Geometry: see drawing. Coordinates: mm, zero at the bounding-box minimum. Round coordinates to 2 decimals unless told otherwise and drop trailing zeros. Order: outer loops, then holes, each group sorted by start corner. A loop starts at its lowest first (then second) coordinate and runs counter-clockwise, first axis right, second up. Notation, with made-up numbers: (16.25, 50) -> (72.25, 50) arc R20 ccw to (72.25, 62) -> close; hole circle Ø8 at (51, -15). An arc over 180 degrees is marked (long way). Use a Markdown table: item, result.
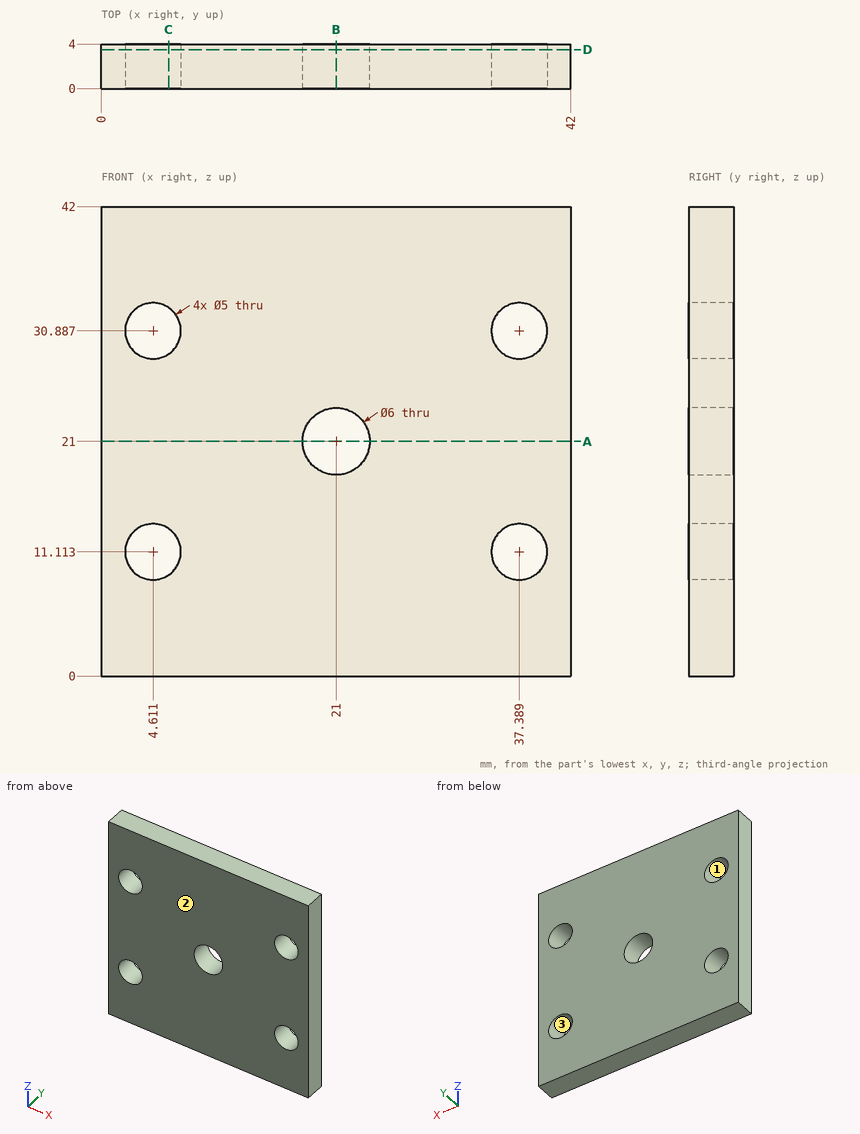
1) Cut plane A-A on z = 21. Return loops of the section in (x, y), and give its area (3 significant figures).
Answer key:
| item | result |
|---|---|
| outline | (0, 0) -> (18, 0) -> (18, 4) -> (0, 4) -> close; (24, 0) -> (42, 0) -> (42, 4) -> (24, 4) -> close |
| area | 144 mm^2 |
2) Draft query along Z for the marked faces 1, 2 and 3. Return one class per face: released by +Z, released by -Z, zero draft, split by the parting line, or undercut.
Answer key:
| item | result |
|---|---|
| face 1 | undercut |
| face 2 | zero draft |
| face 3 | undercut |
3) Cut plane D-D on y = 3.5. Return loops of the section in (x, z), and give its area (3 significant figures).
Answer key:
| item | result |
|---|---|
| outline | (0, 0) -> (42, 0) -> (42, 42) -> (0, 42) -> close; hole circle Ø5 at (4.61, 11.11); hole circle Ø5 at (4.61, 30.89); hole circle Ø6 at (21, 21); hole circle Ø5 at (37.39, 11.11); hole circle Ø5 at (37.39, 30.89) |
| area | 1,660 mm^2 |
4) Cut plane C-C on x = 6. Return loops of the section in (y, z), and give its area (3 significant figures).
Answer key:
| item | result |
|---|---|
| outline | (0, 0) -> (4, 0) -> (4, 9.03) -> (0, 9.03) -> close; (0, 13.19) -> (4, 13.19) -> (4, 28.81) -> (0, 28.81) -> close; (0, 32.97) -> (4, 32.97) -> (4, 42) -> (0, 42) -> close |
| area | 135 mm^2 |
5) Cut plane B-B on x = 21. Return loops of the section in (y, z), and give its area (3 significant figures).
Answer key:
| item | result |
|---|---|
| outline | (0, 0) -> (4, 0) -> (4, 18) -> (0, 18) -> close; (0, 24) -> (4, 24) -> (4, 42) -> (0, 42) -> close |
| area | 144 mm^2 |
6) Ray query, probe 1 along X at (y, z) = (0.25, 11); probe 2 along Z at (x, y) = (4.5, 1.8); probe 3 along X at (y, z) = (3.65, 32.5). Return the intervals inside material, ascending.
Answer key:
| item | result |
|---|---|
| probe 1 | x = 0 to 2.11, 7.11 to 34.89, 39.89 to 42 |
| probe 2 | z = 0 to 8.62, 13.61 to 28.39, 33.38 to 42 |
| probe 3 | x = 0 to 2.7, 6.52 to 35.48, 39.3 to 42 |
